```python
from build123d import *

# Parameters (mm, degrees)
SKETCH1_W           = 33.02
SKETCH1_H           = 22.86
SKETCH1_W_2         = 2.54
SKETCH1_H_2         = 12.7
BOSS_EXTRUDE2_DEPTH = 2.54
SKETCH3_R           = 1.016
BOSS_EXTRUDE3_DEPTH = 2.54
SKETCH4_W           = 33.02
SKETCH4_H           = 22.86
SKETCH4_W_2         = 2.54
SKETCH4_H_2         = 12.7
BOSS_EXTRUDE6_DEPTH = 2.54
SKETCH5_W           = 2.54
SKETCH5_H           = 12.7
BOSS_EXTRUDE7_DEPTH = 2.54


with BuildPart() as part:
    # Sketch1 → Boss-Extrude2 (new body)
    with BuildSketch(Plane(origin=(0, 0, 0), x_dir=(1, 0, 0), z_dir=(0, 1, 0))):
        Rectangle(SKETCH1_W, SKETCH1_H)
        with Locations((-12.74489899, 0)):
            Rectangle(SKETCH1_W_2, SKETCH1_H_2, mode=Mode.SUBTRACT)
        with Locations((12.74489899, 0)):
            Rectangle(SKETCH1_W_2, SKETCH1_H_2, mode=Mode.SUBTRACT)
    extrude(amount=BOSS_EXTRUDE2_DEPTH)

    # Sketch3 → Boss-Extrude3 (add)
    with BuildSketch(Plane(origin=(0, 2.54, 0), x_dir=(1, 0, 0), z_dir=(0, 1, 0))):
        with Locations(Location((-5.318941048, 1.27, 0), (0, 0, 90))):
            Circle(SKETCH3_R)
        with Locations(Location((5.318941048, 1.27, 0), (0, 0, 90))):
            Circle(SKETCH3_R)
    extrude(amount=BOSS_EXTRUDE3_DEPTH)

    # Sketch4 → Boss-Extrude6 (add)
    with BuildSketch(Plane(origin=(0, 5.08, 0), x_dir=(1, 0, 0), z_dir=(0, 1, 0))):
        Rectangle(SKETCH4_W, SKETCH4_H)
        with Locations((-12.74489899, 0)):
            Rectangle(SKETCH4_W_2, SKETCH4_H_2, mode=Mode.SUBTRACT)
        with Locations((12.74489899, 0)):
            Rectangle(SKETCH4_W_2, SKETCH4_H_2, mode=Mode.SUBTRACT)
    extrude(amount=BOSS_EXTRUDE6_DEPTH)

    # Sketch5 → Boss-Extrude7 (add)
    with BuildSketch(Plane(origin=(0, 2.54, 0), x_dir=(1, 0, 0), z_dir=(0, 1, 0))):
        Polygon((-16.51, -11.43), (-16.51, 11.43), (16.51, 11.43), (16.51, -11.43), (10.16, -11.43), (10.16, 6.35), (-10.16, 6.35), (-10.16, -11.43), align=None)
        with Locations((-12.74489899, 0)):
            Rectangle(SKETCH5_W, SKETCH5_H, mode=Mode.SUBTRACT)
        with Locations((12.74489899, 0)):
            Rectangle(SKETCH5_W, SKETCH5_H, mode=Mode.SUBTRACT)
    extrude(amount=BOSS_EXTRUDE7_DEPTH)


solid = part.part
```
Can you work these out from the model? Positions are in its coordinate system, mm. A direction names the side the tool comes from. Round coordinates to 2 decimals unless told otherwise and drop trailing zeros. Loops run counter-clockwise (first coordinate to the right, second up) from the corner with the lowest first, then second, coordinate; pieces in that order, holes last.
Item 1: Please list where these lines run through material, in increasing order: L1, parallel to X at y = 3.75, z = -5.5; L2, parallel to X at y = 1, z = -4.5; L3, parallel to Y at x = 7, z = -0.5.
Item 2: Suppose I cut it at C-C, the plane x = -7. Write out the boundary of the cut face in (y, z).
Item 3: Suppose I cut it at D-D, the plane z = 10. Write out the boundary of the cut face in (x, y), then the cut area to 3 significant figures.
Item 4: If we mould it in two halves opening along X, with no side actions, what happens to faces 1 (the cylindrical face through (-6.326, 3.792, -1.138)), 2 (the flat face through (0, 0, 0)), 3 (the flat face through (16.51, 4, 0))? For each: +X half, -X half, draft (parallel to the pull), parting line (faces both ways), or undercut.
Item 5: Will this pin go through, and if not, where does the flat tip stop? pin 1 Ø1.3 at (x, y) = (-0.5, 4) entering from +Z.
Item 6: Which directions (+Z, -Z, +X, -X, +Y, -Y) give clear straight access to the entire face, cutting with the end or side of a thin tool? Please do faces 4 (the flat face through (-11.475, 4, 0)), 5 (the flat face through (0, 4, -6.35)), 6 (the flat face through (-10.16, 4, 2)).
Item 7: Suppose I cut it at A-A, the plane z = -1.27. Write out the boundary of the cut face in (x, y), then the cut area to 3 significant figures.
Item 8: Suppose I cut it at B-B, the plane y = 1. Write out the boundary of the cut face in (x, z), then the cut area to 3 significant figures.
Reported:
1. L1: x = -16.51 to -14.01, -11.47 to -10.16, 10.16 to 11.47, 14.01 to 16.51
1. L2: x = -16.51 to -14.01, -11.47 to 11.47, 14.01 to 16.51
1. L3: y = 0 to 2.54, 5.08 to 7.62
2. outline: (0, -11.43) - (7.62, -11.43) - (7.62, 11.43) - (5.08, 11.43) - (5.08, -6.35) - (2.54, -6.35) - (2.54, 11.43) - (0, 11.43) - close
3. outline: (-16.51, 0) - (16.51, 0) - (16.51, 7.62) - (-16.51, 7.62) - close; hole (-10.16, 2.54) - (10.16, 2.54) - (10.16, 5.08) - (-10.16, 5.08) - close
3. area: 200 mm2
4. face 1: undercut
4. face 2: draft
4. face 3: +X half
5. pin 1: stops at z = -6.35
6. face 4: +Y, -Y
6. face 5: none
6. face 6: +Z
7. outline: (-16.51, 0) - (-14.01, 0) - (-14.01, 7.62) - (-16.51, 7.62) - close; (-11.47, 0) - (11.47, 0) - (11.47, 7.62) - (-11.47, 7.62) - close; (14.01, 0) - (16.51, 0) - (16.51, 7.62) - (14.01, 7.62) - close; hole (-10.16, 2.54) - (-6.33, 2.54) - (-6.33, 5.08) - (-10.16, 5.08) - close; hole (-4.3, 2.54) - (4.3, 2.54) - (4.3, 5.08) - (-4.3, 5.08) - close; hole (6.33, 2.54) - (10.16, 2.54) - (10.16, 5.08) - (6.33, 5.08) - close
7. area: 172 mm2
8. outline: (-16.51, -11.43) - (16.51, -11.43) - (16.51, 11.43) - (-16.51, 11.43) - close; hole (-14.01, -6.35) - (-11.47, -6.35) - (-11.47, 6.35) - (-14.01, 6.35) - close; hole (11.47, -6.35) - (14.01, -6.35) - (14.01, 6.35) - (11.47, 6.35) - close
8. area: 690 mm2
